Can you work these out from the model? Positions are in its coordinate system, mm. Face numbers are marked on the shaded views. A direction names the side the tool comes from. Round coordinates to 2 decimals unless told otherwise and drop trailing zeros. Write each loop counter-clockwise with the first axis right and the second up, starting at its lowest first coordinate (ties: lowest second). Pieces come first, ordered by that corner, then holes.
Q1. If we section it at A-A (z = 0): Please give me the cut outline in (x, y).
Q2. If we section it at D-D (y = 12.5): Please give me the cut outline in (x, z), plus the area to 3 significant figures.
Q3. I'm going to push flat-ended pins straight in: pin 1 Ø6 at (x, z) = (-4, -4) entering from -Y; pin 2 Ø3 at (y, z) = (8, 4) entering from -X; pin 3 Ø2 at (y, z) = (17.5, -4.5) entering from -X; pin 4 Ø1.2 at (x, z) = (-0.5, -0.5) entering from -Y. Where does each tip first touch, or does it pass through?
Q4. If we section it at B-B (y = 5.75): Please give me the cut outline in (x, z), plus the area to 3 significant figures.
Q5. We'd pull the mould along Z, two halves only. Please class the marked faces 3, 4 and 5: +Z half, -Z half, draft (parallel to the pull), parting line (faces both ways), or undercut.
Q6. If we section it at C-C (x = 0): Please give me the cut outline in (y, z).
Q7. Please list where these lines run through material, in increasing order: line 1 along Z through (x, y) = (-2, 3.5); line 2 along Z through (x, y) = (1.75, 8.5); line 3 along X through (y, z) = (6, 2).
Q8. For the marked faces 1 and 2, which set-ups out of +Z, -Z, +X, -X, +Y, -Y let a thin tool reach every point of the face, with its end or its side?
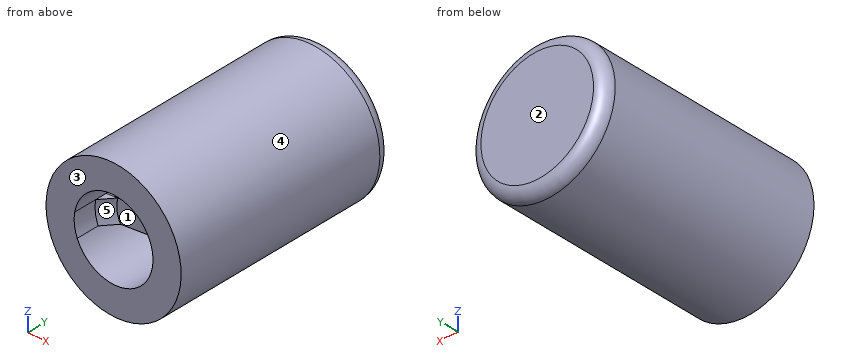
from build123d import *

# Parameters (mm, degrees)
SKETCH1_R           = 6
BOSS_EXTRUDE1_DEPTH = 20
CUT_EXTRUDE1_DEPTH  = 10
CUT_EXTRUDE2_DEPTH  = 3
CHAMFER1_SIZE       = 1
CHAMFER2_SIZE       = 1
FILLET1_R           = 1


with BuildPart() as part:
    # Sketch1 → Boss-Extrude1 (new body)
    with BuildSketch(Plane(origin=(0, 0, 0), x_dir=(1, 0, 0), z_dir=(0, 1, 0))):
        with Locations(Location((0, 0, 0), (0, 0, 270))):
            Circle(SKETCH1_R)
    extrude(amount=BOSS_EXTRUDE1_DEPTH)

    # Sketch2 → Cut-Extrude1 (cut)
    with BuildSketch(Plane.XZ):
        with BuildLine():
            Line((-3.228638435, -1.351256398), (3.447764562, -0.602428024))
            ThreePointArc((3.447764562, -0.602428024), (0.390115429, -3.478190615), (-3.228638435, -1.351256398))
        make_face()
        with BuildLine():
            Line((-3.447764562, 0.602428024), (3.228638435, 1.351256398))
            ThreePointArc((3.228638435, 1.351256398), (-0.390115429, 3.478190615), (-3.447764562, 0.602428024))
        make_face()
    extrude(amount=-CUT_EXTRUDE1_DEPTH, mode=Mode.SUBTRACT)

    # Sketch3 → Cut-Extrude2 (cut)
    with BuildSketch(Plane.XZ):
        with BuildLine():
            Line((-3.447764562, 0.602428024), (3.228638435, 1.351256398))
            ThreePointArc((3.228638435, 1.351256398), (3.478190615, 0.390115429), (3.447764562, -0.602428024))
            Line((3.447764562, -0.602428024), (-3.228638435, -1.351256398))
            ThreePointArc((-3.228638435, -1.351256398), (-3.478190615, -0.390115429), (-3.447764562, 0.602428024))
        make_face()
    extrude(amount=-CUT_EXTRUDE2_DEPTH, mode=Mode.SUBTRACT)

    # Chamfer1
    chamfer1_edges = [part.edges().sort_by_distance(p)[0] for p in [
        (-0.390115429, 10, 3.478190615),
        (-0.109563063, 10, 0.976842211),
        (0.390115429, 10, -3.478190615),
        (0.109563063, 10, -0.976842211),
    ]]
    chamfer(chamfer1_edges, length=CHAMFER1_SIZE)

    # Chamfer2
    # the kernel refuses this chamfer: 1 mm, written as the material it adds along each edge
    with BuildSketch(Plane(origin=(0, 3, 0), x_dir=(-0.42559561828763903, 0, -0.9049134597818524), z_dir=(0.9049134597818524, 0, -0.42559561828763903))) as chamfer2_piece_1_section:
        Polygon((3.5, -CHAMFER2_SIZE), (3.5 - CHAMFER2_SIZE, 0), (3.5, 0), align=None)
    chamfer2_piece_1 = revolve(axis=Axis((0, 3, 0), (0, 1, 0)), revolution_arc=116.82411124, mode=Mode.PRIVATE)
    chamfer2_piece_1 = split(chamfer2_piece_1, bisect_by=Plane(origin=(-2.987774237, 2.670615871, -1.324240961), z_dir=(-0.11146155122457255, 0, 0.9937687470425964)), keep=Keep.TOP, mode=Mode.PRIVATE)
    chamfer2_piece_1 = split(chamfer2_piece_1, bisect_by=Plane(origin=(-3.206900364, 2.670615871, 0.629443462), z_dir=(0.11146155122457255, 0, -0.9937687470425964)), keep=Keep.TOP, mode=Mode.PRIVATE)
    add(chamfer2_piece_1)
    with BuildSketch(Plane(origin=(0, 3, 0), x_dir=(0.4255956182876634, 0, 0.904913459781841), z_dir=(-0.904913459781841, 0, 0.4255956182876634))) as chamfer2_piece_2_section:
        Polygon((3.5, -CHAMFER2_SIZE), (3.5 - CHAMFER2_SIZE, 0), (3.5, 0), align=None)
    chamfer2_piece_2 = revolve(axis=Axis((0, 3, 0), (0, 1, 0)), revolution_arc=116.82411124, mode=Mode.PRIVATE)
    chamfer2_piece_2 = split(chamfer2_piece_2, bisect_by=Plane(origin=(3.206900364, 2.670615871, -0.629443462), z_dir=(-0.11146155122457255, 0, 0.9937687470425964)), keep=Keep.TOP, mode=Mode.PRIVATE)
    chamfer2_piece_2 = split(chamfer2_piece_2, bisect_by=Plane(origin=(2.987774237, 2.670615871, 1.324240961), z_dir=(0.11146155122457255, 0, -0.9937687470425964)), keep=Keep.TOP, mode=Mode.PRIVATE)
    add(chamfer2_piece_2)

    # Fillet1
    fillet1_edges = [part.edges().sort_by_distance(p)[0] for p in [
        (0, 20, -6),
    ]]
    fillet(fillet1_edges, radius=FILLET1_R)


solid = part.part
A:
1. outline: (-6, 0) - (-3.5, 0) - (-3.5, 2) - (-2.5, 3) - (2.5, 3) - (3.5, 2) - (3.5, 0) - (6, 0) - (6, 19) arc R1 ccw to (5, 20) - (-5, 20) arc R1 ccw to (-6, 19) - close
2. outline: circle Ø12 at (0, 0)
2. area: 113 mm2
3. pin 1: stops at y = 0
3. pin 2: stops at x = -5.45
3. pin 3: stops at x = -4.87
3. pin 4: stops at y = 3
4. outline: circle Ø12 at (0, 0); hole (-3.45, 0.6) - (3.23, 1.35) arc R3.5 ccw to start; hole (-3.23, -1.35) arc R3.5 ccw to (3.45, -0.6) - close
4. area: 88.2 mm2
5. face 3: draft
5. face 4: parting line
5. face 5: undercut
6. outline: (0, -6) - (19, -6) arc R1 ccw to (20, -5) - (20, 5) arc R1 ccw to (19, 6) - (0, 6) - (0, 3.5) - (9, 3.5) - (10, 2.5) - (10, 2) - (9, 0.99) - (3, 0.99) - (3, -0.99) - (9, -0.99) - (10, -2) - (10, -2.5) - (9, -3.5) - (0, -3.5) - close
7. line 1: z = -5.66 to -2.87, -1.21 to 0.76, 2.87 to 5.66
7. line 2: z = -5.74 to -3.03, -0.79 to 1.19, 3.03 to 5.74
7. line 3: x = -5.66 to -2.87, 2.87 to 5.66
8. face 1: -Y
8. face 2: +Z, -Z, +X, -X, +Y
